For this review, use the dimensioned drawing (mm, ordinates from the lowest corner) and the shaded views. Round coordinates to 2 decimals unless told otherwise and drop trailing zeros. Loops run counter-clockwise (first coordinate to the right, second up) from the corner with the lowest first, then second, coordinate; pieces in that order, holes last. Notation, with made-up numbers: (-36.75, 72.25) -> (-17.75, 72.25) arc R12 cw to (-17.75, 80.25) -> close; hole circle Ø7 at (66.25, 32). An arc over 180 degrees is marked (long way). Answer as CSV lines item,"result". Start each with the question number.
(1) Take a section at D-D, the plane x = 35. Write out the cut boundary in (y, z).
(2) Take a section at B-B, the plane x = 79.5. Write out the cut boundary in (y, z).
(3) Take a section at C-C, the plane z = 1.5. Write out the cut boundary in (x, y) (1 decimal), and give its area (3 significant figures).
(4) To check wall thickness, follow line 1 (Y direction, x = 66.5, z = 3); line 2 (Y direction, x = 35.5, z = 4); line 3 (X direction, y = 47, z = 4.75). State the ranges of each line that lie inside material, in increasing order. Write a range as from..to.
(5) Take a section at A-A, the plane y = 43.5. Write out the cut boundary in (x, z), and give its area (3 significant figures).
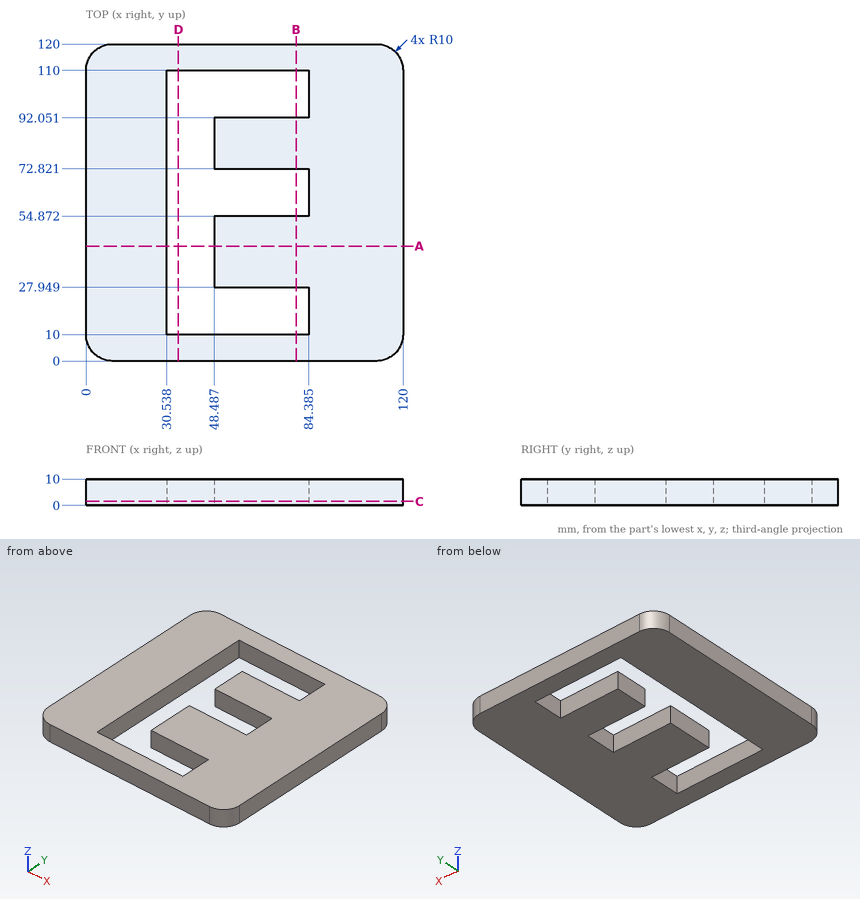
The answers:
1,outline,"(0, 0) -> (10, 0) -> (10, 10) -> (0, 10) -> close; (110, 0) -> (120, 0) -> (120, 10) -> (110, 10) -> close"
2,outline,"(0, 0) -> (10, 0) -> (10, 10) -> (0, 10) -> close; (27.95, 0) -> (54.87, 0) -> (54.87, 10) -> (27.95, 10) -> close; (72.82, 0) -> (92.05, 0) -> (92.05, 10) -> (72.82, 10) -> close; (110, 0) -> (120, 0) -> (120, 10) -> (110, 10) -> close"
3,outline,"(0, 10) arc R10 ccw to (10, 0) -> (110, 0) arc R10 ccw to (120, 10) -> (120, 110) arc R10 ccw to (110, 120) -> (10, 120) arc R10 ccw to (0, 110) -> close; hole (30.5, 10) -> (84.4, 10) -> (84.4, 27.9) -> (48.5, 27.9) -> (48.5, 54.9) -> (84.4, 54.9) -> (84.4, 72.8) -> (48.5, 72.8) -> (48.5, 92.1) -> (84.4, 92.1) -> (84.4, 110) -> (30.5, 110) -> close"
3,area,"10,600 mm²"
4,line 1,"0..10, 27.95..54.87, 72.82..92.05, 110..120"
4,line 2,"0..10, 110..120"
4,line 3,"0..30.54, 48.49..120"
5,outline,"(0, 0) -> (30.54, 0) -> (30.54, 10) -> (0, 10) -> close; (48.49, 0) -> (120, 0) -> (120, 10) -> (48.49, 10) -> close"
5,area,"1,020 mm²"
